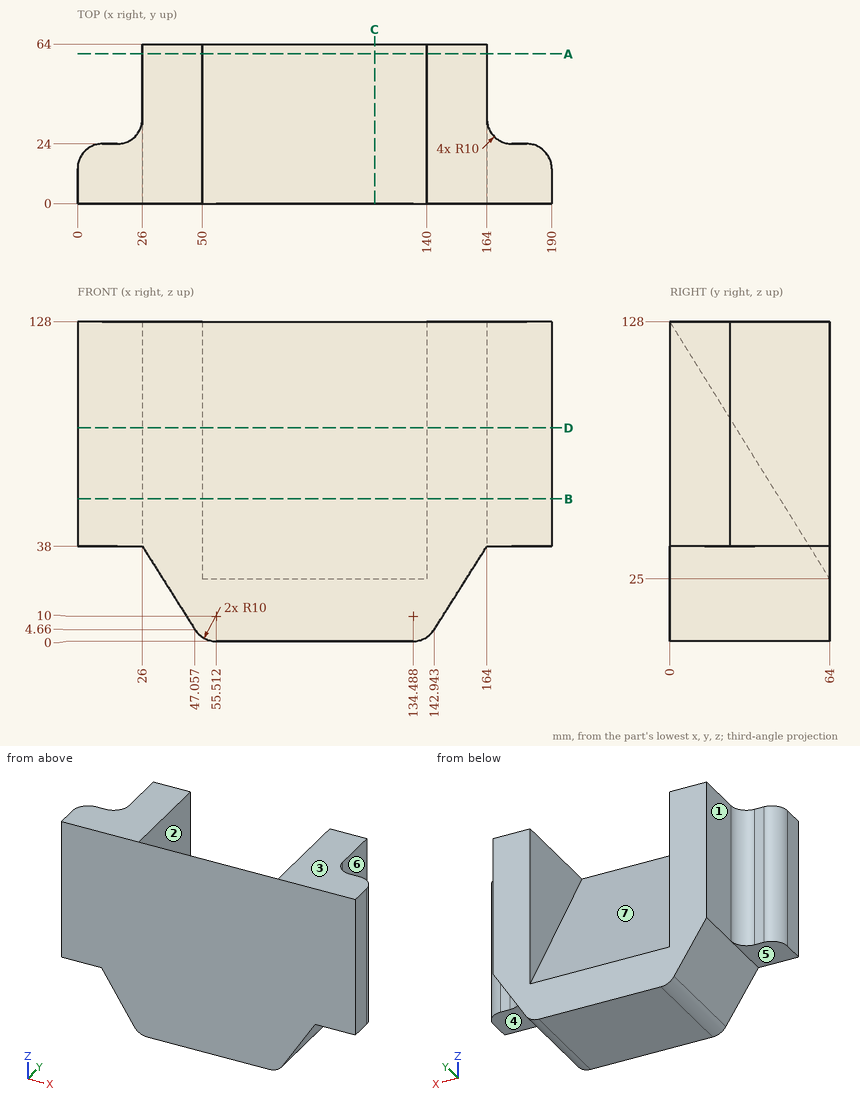
Part print with two shaded views. Sizes in mm from the minimum x, y, z corner. A direction names the side the tool comes from. Give positions to 0.01 mm unless a question says otherwise; leave off trailing zeros. Loops run counter-clockwise (first coordinate to the right, second up) from the corner with the lowest first, then second, coordinate; pieces in that order, holes last. Notation, with made-up numbers: (53, 38) - (88, 38) arc R16 ccw to (88, 67) - close; hole circle Ø8 at (40.25, -31). An arc over 180 degrees is marked (long way). Put each result on its own line as item: value.
Q1. Slice it at C-C (x = 119). Give the cut face in (y, z).
Filled in:
outline: (0, 0) - (64, 0) - (64, 25) - (0, 128) - close
Q2. Flat gauge pins, fed straight in: pin 1 (24 mm diameter, centred on y = 43.5, z = 95.5, fed in from -X); pin 2 (1.8 mm diameter, centred on x = 178, z = 78.5, fed in from +Y); pin 3 (12 mm diameter, centred on y = 27, z = 48, fed in from +X). Where does each tip first touch, or does it go through?
Filled in:
pin 1: stops at x = 25.68
pin 2: stops at y = 24
pin 3: stops at x = 187.14
Q3. Slice it at B-B (z = 57). Give the cut face in (x, y).
Filled in:
outline: (0, 0) - (190, 0) - (190, 14) arc R10 ccw to (180, 24) - (174, 24) arc R10 cw to (164, 34) - (164, 64) - (140, 64) - (140, 44.12) - (50, 44.12) - (50, 64) - (26, 64) - (26, 34) arc R10 cw to (16, 24) - (10, 24) arc R10 ccw to (0, 14) - close
Q4. Probe line 1 along X through (y, z) = (58.5, 103.5); line 2 along Y through (x, z) = (174, 122); line 3 along X through (y, z) = (41, 52.5). List the from-to ranges inside material, lowest first.
Filled in:
line 1: x = 26 to 50, 140 to 164
line 2: y = 0 to 24
line 3: x = 26 to 164
Q5. Slice it at A-A (y = 60). Give the cut face in (x, z).
Filled in:
outline: (26, 38) - (47.06, 4.66) arc R10 ccw to (55.51, 0) - (134.49, 0) arc R10 ccw to (142.94, 4.66) - (164, 38) - (164, 128) - (140, 128) - (140, 31.44) - (50, 31.44) - (50, 128) - (26, 128) - close
Q6. Mould opens along X. For the marked faces 1, 2 and 3 say: pulls with the +X half, pulls with the -X half, needs draft (parallel to the pull), parting line crosses it, or undercut.
Filled in:
face 1: pulls with the -X half
face 2: undercut
face 3: needs draft
Q7. Tool access for the marked faces 4, 5, 6 and 7: list every direction of +Z, -Z, +X, -X, +Y, -Y with a clear straight run to the whole face (end or side of a thin tool).
Filled in:
face 4: -Z, +X, +Y, -Y
face 5: -Z, -X, +Y, -Y
face 6: +Z, -Z, +X, +Y
face 7: +Z, +Y
Q8. Slice it at D-D (z = 85.5). Give the cut face in (x, y), plus the area to 3 significant figures.
Filled in:
outline: (0, 0) - (190, 0) - (190, 14) arc R10 ccw to (180, 24) - (174, 24) arc R10 cw to (164, 34) - (164, 64) - (140, 64) - (140, 26.41) - (50, 26.41) - (50, 64) - (26, 64) - (26, 34) arc R10 cw to (16, 24) - (10, 24) arc R10 ccw to (0, 14) - close
area: 6,700 mm²
